```python
from build123d import *

# Parameters (mm, degrees)
SKETCH1_R           = 5
BOSS_EXTRUDE1_DEPTH = 3
BOSS_EXTRUDE2_DEPTH = 3
CIRPATTERN2_COUNT   = 7
SKETCH3_R           = 4.5
CUT_EXTRUDE1_DEPTH  = 0.1
SKETCH4_R           = 1.5
BOSS_EXTRUDE3_DEPTH = 1
SKETCH5_R           = 0.75
CUT_EXTRUDE2_DEPTH  = 12.937398013


with BuildPart() as part:
    # Sketch1 → Boss-Extrude1 (new body)
    with BuildSketch(Plane.XY):
        Circle(SKETCH1_R)
    extrude(amount=BOSS_EXTRUDE1_DEPTH)

    # Sketch2 → Boss-Extrude2 (add)
    with BuildSketch(Plane.XY.offset(3)):
        with BuildLine():
            Line((-1.46243537, 4.781347382), (1.46243537, 4.781347382))
            Line((1.46243537, 4.781347382), (0.6, 8))
            ThreePointArc((0.6, 8), (0, 8.022468448), (-0.6, 8))
            Line((-0.6, 8), (-1.46243537, 4.781347382))
        make_face()
    boss_extrude2 = extrude(amount=-BOSS_EXTRUDE2_DEPTH)

    # CirPattern2: Boss-Extrude2 ×7 about axis
    cirpattern2_axis = Axis((0, 0, 0), (0, 0, 1))
    for i in range(1, CIRPATTERN2_COUNT):
        add(boss_extrude2.rotate(cirpattern2_axis, i * 360 / CIRPATTERN2_COUNT))

    # Sketch3 → Cut-Extrude1 (cut)
    with BuildSketch(Plane.XY.offset(3)):
        Circle(SKETCH3_R)
    extrude(amount=-CUT_EXTRUDE1_DEPTH, mode=Mode.SUBTRACT)

    # Sketch4 → Boss-Extrude3 (add)
    with BuildSketch(Plane.XY.offset(2.9)):
        Circle(SKETCH4_R)
    extrude(amount=BOSS_EXTRUDE3_DEPTH)

    # Sketch5 → Cut-Extrude2 (cut, through all)
    with BuildSketch(Plane.XY.offset(3.9)):
        Circle(SKETCH5_R)
    extrude(amount=-CUT_EXTRUDE2_DEPTH, mode=Mode.SUBTRACT)


solid = part.part
```
Geometry check sheet. Reference: the model listing, model coordinates, mm. A direction names the side the tool comes from. Round coordinates to 2 decimals unless told otherwise and drop trailing zeros. Loops run counter-clockwise (first coordinate to the right, second up) from the corner with the lowest first, then second, coordinate; pieces in that order, holes last. Notation, with made-up numbers: M 31.25,-24 L 85.25,-24 A6 cw 85.25,-15 Z; hole C 30,25.25 d11. An arc over 180 degrees is marked long. Return JSON: item names as keys, results as strings. Group by question number.
(1) Scan lines: line 1 along Y through (x, z) = (0, 2.95); line 2 along Y through (x, z) = (0, 3.05); line 3 along Y through (x, z) = (0, 1.9). Record each from-to range of solid material in increasing order. Write a range as [from, to].
(2) Go/stop test with flat-tipped pins: pin 1 (2 mm diameter, centred on x = -5.5, z = 0.5, fed in from -Y); pin 2 (1.5 mm diameter, centred on x = 1.5, z = 1.5, fed in from -Y); pin 3 (1.4 mm diameter, centred on x = 0, y = 0, fed in from +Z); pin 4 (6 mm diameter, centred on x = 4, y = -3.5, fed in from -Z). Record where each tip stops, or that it passes through.
(3) Section check D-D, the plane x = 2.25. Enter the section's corners in (y, z), and give its area (3 significant figures).
(4) Section check C-C, the plane y = 0. Enter the section's corners in (x, z), and give its area (3 significant figures).
(5) Section check B-B, the plane x = 0. Enter the section's corners in (y, z).
(6) Mould release check, pull along X, two halves, no side actions. Record for faces 1 (the face through (7.82, -1.79, 1.52)), 2 (the face through (-5.653, 3.197, 1.521)), 3 (the face through (-4.33, 4.78, 1.52)): pulls with the +X half, pulls with the -X half, needs draft (parallel to the pull), parting line crosses it, or undercut.
(7) Set-up check for faces 4 (the face through (4, -3, 1)), 5 (the face through (-1.5, 0.07, 3.39)), 6 (the face through (-3.7, -5.3, 1.5)), 7 (the face through (-1.025, 6.413, 1.521)), 8 (the face through (-1.859, -6.223, 1.521)): record each of +Z, -Z, +X, -X, +Y, -Y from which the full face is reachable in a straight line by a thin tool's end or side.
Data:
{
 "1": {"line 1": "[-5, -4.5], [-1.5, -0.75], [0.75, 1.5], [4.5, 8.02]", "line 2": "[-1.5, -0.75], [0.75, 1.5]", "line 3": "[-5, -0.75], [0.75, 8.02]"},
 "2": {"pin 1": "y = -2.48", "pin 2": "y = -6.68", "pin 3": "through", "pin 4": "z = 0"},
 "3": {"outline": "M -6.68,0 L 4.47,0 L 4.47,3 L 3.9,3 L 3.9,2.9 L -3.9,2.9 L -3.9,3 L -6.68,3 Z", "area": "32.6 mm²"},
 "4": {"outline": "M -5.67,0 L -0.75,0 L -0.75,3.9 L -1.5,3.9 L -1.5,2.9 L -4.5,2.9 L -4.5,3 L -5.67,3 Z; M 0.75,0 L 5.67,0 L 5.67,3 L 4.5,3 L 4.5,2.9 L 1.5,2.9 L 1.5,3.9 L 0.75,3.9 Z", "area": "30.3 mm²"},
 "5": {"outline": "M -5,0 L -0.75,0 L -0.75,3.9 L -1.5,3.9 L -1.5,2.9 L -4.5,2.9 L -4.5,3 L -5,3 Z; M 0.75,0 L 8.02,0 L 8.02,3 L 4.5,3 L 4.5,2.9 L 1.5,2.9 L 1.5,3.9 L 0.75,3.9 Z"},
 "6": {"face 1": "pulls with the +X half", "face 2": "pulls with the -X half", "face 3": "undercut"},
 "7": {"face 4": "+Z, -Z, +X", "face 5": "+Z", "face 6": "+Z, -Z, -X", "face 7": "+Z, -Z, +Y", "face 8": "+Z, -Z, -Y"}
}
